```python
from build123d import *

# Parameters (mm, degrees)
BOSS_EXTRUDE1_DEPTH = 2
CIRPATTERN1_COUNT   = 4
SKETCH2_R           = 1.5
SKETCH2_R_2         = 2
CUT_EXTRUDE1_DEPTH  = 2
CUT_EXTRUDE2_DEPTH  = 2
FILLET2_R           = 1


with BuildPart() as part:
    # Sketch1 → Boss-Extrude1 (new body)
    with BuildSketch(Plane(origin=(0, 0, 0), x_dir=(1, 0, 0), z_dir=(0, 1, 0))):
        with BuildLine():
            Line((0, 25), (0, 0))
            Line((0, 0), (25, 0))
            ThreePointArc((25, 0), (23.535533906, 3.535533906), (20, 5))
            ThreePointArc((20, 5), (9.393398282, 9.393398282), (5, 20))
            ThreePointArc((5, 20), (3.535533906, 23.535533906), (0, 25))
        make_face()
    boss_extrude1 = extrude(amount=BOSS_EXTRUDE1_DEPTH)

    # CirPattern1: Boss-Extrude1 ×4 about axis
    cirpattern1_axis = Axis((0, 0, 0), (0, 1, 0))
    for i in range(1, CIRPATTERN1_COUNT):
        add(boss_extrude1.rotate(cirpattern1_axis, i * 360 / CIRPATTERN1_COUNT))

    # Sketch2 → Cut-Extrude1 (cut)
    with BuildSketch(Plane(origin=(0, 2, 0), x_dir=(1, 0, 0), z_dir=(0, 1, 0))):
        with Locations(Location((0, 11.313708499, 0), (0, 0, 270))):
            Circle(SKETCH2_R)
        with Locations(Location((0, 20, 0), (0, 0, 270))):
            Circle(SKETCH2_R_2)
        with Locations(Location((11.313708499, 0, 0), (0, 0, 270))):
            Circle(SKETCH2_R)
        with Locations(Location((20, 0, 0), (0, 0, 270))):
            Circle(SKETCH2_R_2)
        with Locations(Location((0, -11.313708499, 0), (0, 0, 270))):
            Circle(SKETCH2_R)
        with Locations(Location((0, -20, 0), (0, 0, 270))):
            Circle(SKETCH2_R_2)
        with Locations(Location((-11.313708499, 0, 0), (0, 0, 270))):
            Circle(SKETCH2_R)
        with Locations(Location((-20, 0, 0), (0, 0, 270))):
            Circle(SKETCH2_R_2)
    extrude(amount=-CUT_EXTRUDE1_DEPTH, mode=Mode.SUBTRACT)

    # Sketch3 → Cut-Extrude2 (cut)
    with BuildSketch(Plane(origin=(0, 2, 0), x_dir=(1, 0, 0), z_dir=(0, 1, 0))):
        with BuildLine():
            Line((-11.212704416, 2.929431208), (-2.929431208, 11.212704416))
            ThreePointArc((-2.929431208, 11.212704416), (0, 8.859568233), (2.929431208, 11.212704416))
            Line((2.929431208, 11.212704416), (11.212704416, 2.929431208))
            ThreePointArc((11.212704416, 2.929431208), (8.859568233, 0), (11.212704416, -2.929431208))
            Line((11.212704416, -2.929431208), (2.929431208, -11.212704416))
            ThreePointArc((2.929431208, -11.212704416), (0, -8.859568233), (-2.929431208, -11.212704416))
            Line((-2.929431208, -11.212704416), (-11.212704416, -2.929431208))
            ThreePointArc((-11.212704416, -2.929431208), (-8.859568233, 0), (-11.212704416, 2.929431208))
        make_face()
    extrude(amount=-CUT_EXTRUDE2_DEPTH, mode=Mode.SUBTRACT)

    # Fillet2
    fillet2_edges = [part.edges().sort_by_distance(p)[0] for p in [
        (-11.212704416, 1, 2.929431208),
        (-11.212704416, 1, -2.929431208),
        (-2.929431208, 1, -11.212704416),
        (2.929431208, 1, -11.212704416),
        (11.212704416, 1, -2.929431208),
        (11.212704416, 1, 2.929431208),
        (2.929431208, 1, 11.212704416),
        (-2.929431208, 1, 11.212704416),
    ]]
    fillet(fillet2_edges, radius=FILLET2_R)


solid = part.part
```
For this review, take the finished solid that the model builds, in its own axes (mm). A direction names the side the tool comes from. Coordinates: 2 decimals unless noted, no trailing zeros. Write each loop counter-clockwise with the first axis right and the second up, starting at its lowest first coordinate (ties: lowest second). Pieces come first, ordered by that corner, then holes. Notation, with made-up numbers: (6.25, -39.5) - (52.25, -39.5) arc R16 ccw to (52.25, -9.5) - close; hole circle Ø4 at (72.25, 67.25). An arc over 180 degrees is marked (long way). Answer in a Markdown table with one row per item. Add a question column.
Q1. We need section B-B, the plane x = -8. State the section outline as (y, z) points.
Q2. We need section C-C, the plane y = 1.45. Count the separate pieces of the cut face and the enclosed holes in it, and give its area (3 significant figures).
Q3. Tool access review of faces 1 (the cylindrical face through (-8.86, 1.01, 0.04)), 2 (the flat face through (0.1, 2, -9.4)): name each direction out of +Z, -Z, +X, -X, +Y, -Y from which nothing blocks a thin tool from reaching the whole face with its end or side.
Q4. For P1, Ø1, axis at x = -3, y = 0.5, coming from the -Z side, flat-tipped, find the tip position at first contact; note if it passes through.
Q5. Draft analysis for pull direction X (two halves, no side actions). For faces 3 (the flat face through (0.1, 0, -9.4)), 4 (the cylindrical face through (-9.28, 0.99, -9.51)), 5 (the cylindrical face through (0.066, 1.014, 9.815)), state which applies: +X half, -X half, draft (parallel to the pull), parting line (faces both ways), or undercut.
Q6. We need section A-A, the plane x = 3. State the section outline as (y, z) points, and give its area (3 significant figures).
Q7. For probe 1 along X at (y, z) = (0.95, 20); probe 2 along X at (y, z) = (0.6, 4); probe 3 along Z at (x, y) = (12, 1.85), list the stretches that pass through material, from the lowest coordinate up.
Answer list:
| question | item | result |
|---|---|---|
| 1 | outline | (0, -11) - (2, -11) - (2, -6.14) - (0, -6.14) - close; (0, 6.14) - (2, 6.14) - (2, 11) - (0, 11) - close |
| 2 | separate pieces | 1 |
| 2 | enclosed holes | 9 |
| 2 | area | 650 mm2 |
| 3 | face 1 | +Y, -Y |
| 3 | face 2 | +Z, -Z, +X, -X, +Y |
| 4 | P1 | stops at z = -24.33 |
| 5 | face 3 | draft |
| 5 | face 4 | -X half |
| 5 | face 5 | undercut |
| 6 | outline | (0, -24) - (2, -24) - (2, -10.47) - (0, -10.47) - close; (0, 10.47) - (2, 10.47) - (2, 24) - (0, 24) - close |
| 6 | area | 54.1 mm2 |
| 7 | probe 1 | x = -5 to -2, 2 to 5 |
| 7 | probe 2 | x = -23 to -10.14, 10.14 to 23 |
| 7 | probe 3 | z = -7.31 to -1.33, 1.33 to 7.31 |
